```python
from build123d import *

# Parameters (mm, degrees)
SKETCH1_W           = 30
SKETCH1_H           = 45
BOSS_EXTRUDE1_DEPTH = 5
SKETCH2_R           = 1.95
SKETCH2_W           = 21.5
SKETCH2_H           = 34.25
CUT_EXTRUDE1_DEPTH  = 6
SKETCH3_W           = 15
SKETCH3_H           = 4
BOSS_EXTRUDE2_DEPTH = 6
SKETCH4_R           = 1.55
CUT_EXTRUDE2_DEPTH  = 5


with BuildPart() as part:
    # Sketch1 → Boss-Extrude1 (new body)
    with BuildSketch(Plane(origin=(0, 0, 0), x_dir=(1, 0, 0), z_dir=(0, 1, 0))):
        Rectangle(SKETCH1_W, SKETCH1_H)
    extrude(amount=BOSS_EXTRUDE1_DEPTH)

    # Sketch2 → Cut-Extrude1 (cut, through all)
    with BuildSketch(Plane(origin=(0, 5, 0), x_dir=(1, 0, 0), z_dir=(0, 1, 0))):
        with Locations((10.75, 19)):
            Circle(SKETCH2_R)
        with Locations((10.75, -16)):
            Circle(SKETCH2_R)
        with Locations((-10.75, -16)):
            Circle(SKETCH2_R)
        with Locations((-4.25, 5.375)):
            Rectangle(SKETCH2_W, SKETCH2_H)
    extrude(amount=-CUT_EXTRUDE1_DEPTH, mode=Mode.SUBTRACT)

    # Sketch3 → Boss-Extrude2 (add)
    with BuildSketch(Plane(origin=(0, 5, 0), x_dir=(1, 0, 0), z_dir=(0, 1, 0))):
        with Locations((0, -20.5)):
            Rectangle(SKETCH3_W, SKETCH3_H)
    extrude(amount=BOSS_EXTRUDE2_DEPTH)

    # Sketch4 → Cut-Extrude2 (cut, through all)
    with BuildSketch(Plane(origin=(0, 0, 18.5), x_dir=(-1, 0, 0), z_dir=(0, 0, -1))):
        with Locations((-5, 8)):
            Circle(SKETCH4_R)
        with Locations((5, 8)):
            Circle(SKETCH4_R)
    extrude(amount=-CUT_EXTRUDE2_DEPTH, mode=Mode.SUBTRACT)


solid = part.part
```
The listing builds one solid part. Answer for the finished solid, in the listing's coordinates (mm). A direction names the side the tool comes from. Round coordinates to 2 decimals unless told otherwise and drop trailing zeros. Loops run counter-clockwise (first coordinate to the right, second up) from the corner with the lowest first, then second, coordinate; pieces in that order, holes last. Notation, with made-up numbers: (51.5, 80.25) - (63.5, 80.25) arc R18 cw to (63.5, 93.25) - close; hole circle Ø4 at (66.5, -27.75). An arc over 180 degrees is marked (long way). Use one line per item in the form item = value. Start each with the question number.
1. The part is cut by section C-C on y = 8. Determine the outline of the cut face in (x, z).
2. The part is cut by section A-A on x = -5. Determine the outline of the cut face in (y, z).
3. Given pin 1 Ø2.5 at (x, y) = (-3.5, 2.5) entering from -Z; pin 2 Ø2.5 at (x, z) = (10.75, 16) entering from -Y; pin 3 Ø1.5 at (x, y) = (-4.5, 9) entering from -Z; pin 4 Ø1 at (x, z) = (6.5, -12) entering from +Y, each flat-ended and moving along its own axis, determine where each tip first touches the part or whether it passes through.
4. Consider line 1 (X direction, y = 1.45, z = 16); line 2 (Z direction, x = 10.75, y = 3.4); line 3 (Y direction, x = 5, z = 20.15). Determine where each line is inside the solid, lowest interval first. Write a range as [from, to].
5. The part is cut by section B-B on z = -19. Determine the outline of the cut face in (x, y), then the cut area to 3 significant figures.
6. A tool of negligible diameter and unlimited length cuts with its end or side. For faces 1 (the face through (6.5, 3, -5)), 2 (the face through (0, 8, 18.5)), 3 (the face through (7.5, 8, 21)), from which of +Z, -Z, +X, -X, +Y, -Y can it reach the whole face along a straight path? Write none if from no direction.
7. The part is cut by section D-D on x = 10.75. Determine the outline of the cut face in (y, z).
8. For a pull along Y with two mould halves and no side action, classify faces 4 (the face through (0, 11, 20)), 5 (the face through (-3.45, 8.07, 20.47)), 6 (the face through (-7.5, 8, 21)) as pulls with the +Y half, pulls with the -Y half, needs draft (parallel to the pull), parting line crosses it, or undercut.
Geometry check:
q1.outline = (-7.5, 18.5) - (-6.55, 18.5) - (-6.55, 22.5) - (-7.5, 22.5) - close; (-3.45, 18.5) - (3.45, 18.5) - (3.45, 22.5) - (-3.45, 22.5) - close; (6.55, 18.5) - (7.5, 18.5) - (7.5, 22.5) - (6.55, 22.5) - close
q2.outline = (0, 11.75) - (5, 11.75) - (5, 18.5) - (6.45, 18.5) - (6.45, 22.5) - (0, 22.5) - close; (9.55, 18.5) - (11, 18.5) - (11, 22.5) - (9.55, 22.5) - close
q3.pin_1 = 11.75
q3.pin_2 = through
q3.pin_3 = 18.5
q3.pin_4 = 5
q4.line_1 = [-15, -12.7], [-8.8, 8.8], [12.7, 15]
q4.line_2 = [-22.5, -20.95], [-17.05, 14.05], [17.95, 22.5]
q4.line_3 = [0, 6.45], [9.55, 11]
q5.outline = (6.5, 0) - (8.8, 0) - (8.8, 5) - (6.5, 5) - close; (12.7, 0) - (15, 0) - (15, 5) - (12.7, 5) - close
q5.area = 23.0 mm^2
q6.face_1 = -Z, -X, +Y, -Y
q6.face_2 = -Z, +X, -X, +Y
q6.face_3 = +Z, -Z, +X, +Y
q7.outline = (0, -22.5) - (5, -22.5) - (5, -20.95) - (0, -20.95) - close; (0, -17.05) - (5, -17.05) - (5, 14.05) - (0, 14.05) - close; (0, 17.95) - (5, 17.95) - (5, 22.5) - (0, 22.5) - close
q8.face_4 = pulls with the +Y half
q8.face_5 = undercut
q8.face_6 = needs draft
